from build123d import *

# Parameters (mm, degrees)
F1_DEPTH = 25.4


with BuildPart() as f1:
    # F0 (on Front) → F1 (new body)
    with BuildSketch(Plane.XZ):
        Polygon((47.539182, 77.96976), (47.539182, 65.957407), (47.539182, 61.33727), (47.539182, 53.945053), (91.276467, 53.945053), (91.276467, 77.96976), align=None)
        with BuildLine():
            Line((-2.96659, 32.384418), (-2.96659, 19.140026))
            Line((-2.96659, 19.140026), (15.205946, 19.140026))
            Line((15.205946, 19.140026), (15.205946, 42.856727))
            ThreePointArc((15.205946, 42.856727), (26.010861, 61.477741), (47.539182, 61.33727))
            Line((47.539182, 61.33727), (47.539182, 65.957407))
            ThreePointArc((47.539182, 65.957407), (13.287985, 62.707588), (-2.96659, 32.384418))
        make_face()
        Polygon((-2.96659, 19.140026), (-31.311143, 19.140026), (-31.311143, -19.140026), (31.311143, -19.140026), (31.311143, 19.140026), (15.205946, 19.140026), align=None)
    extrude(amount=F1_DEPTH)


solid = f1.part
Could you check a few things on this model? Use its own coordinates, in mm. A direction names the side the tool comes from. Round coordinates to 2 decimals unless told otherwise and drop trailing zeros. Order: outer loops, then holes, each group sorted by start corner. A loop starts at its lowest first (then second) coordinate and runs counter-clockwise, first axis right, second up.
(1) Please list where these lines run through material, in increasing order: line 1 along Z through (x, y) = (-15.5, -6.5); line 2 along X through (y, z) = (-19.75, 11.5); line 3 along Z through (x, y) = (28, -8.5).
Response values:
line 1: z = -19.14 to 19.14
line 2: x = -31.31 to 31.31
line 3: z = -19.14 to 19.14, 62.48 to 68.39
(2) If we mould it in two halves opening along X, with no side actions, what happens to faces 6 (the flat face through (-31.311, -13, 0)), 7 (the flat face through (-17, -13, 19.14)), 8 (the cylindrical face through (13.708, -12.522, 62.982)), 9 (the flat face through (47.539, -13, 72))? For each: released by +X, released by -X, zero draft, split by the parting line, or undercut.
Response values:
face 6: released by -X
face 7: zero draft
face 8: undercut
face 9: undercut
(3) Imagine slicing it at D-D (x = 53.5). Write out the boundary of the cut face in (y, z).
Response values:
outline: (-25.4, 53.95) - (0, 53.95) - (0, 77.97) - (-25.4, 77.97) - close
(4) Imagine slicing it at C-C (z = 55.5). Write out the boundary of the cut face in (x, y).
Response values:
outline: (5.31, -25.4) - (19.33, -25.4) - (19.33, 0) - (5.31, 0) - close; (47.54, -25.4) - (91.28, -25.4) - (91.28, 0) - (47.54, 0) - close
(5) I'm going to push flat-ended pins straight in: pin 1 (1 mm diameter, centred on x = 34, y = -5.5, fed in from +Z); pin 2 (7.5 mm diameter, centred on x = -24, y = -8.5, fed in from +Z); pin 3 (4 mm diameter, centred on y = -15, z = 27.5, fed in from -X); pin 4 (12 mm diameter, centred on x = 2, z = 7.5, fed in from +Y). Where does each tip first touch, or does it pass through?
Response values:
pin 1: stops at z = 68.8
pin 2: stops at z = 19.14
pin 3: stops at x = -2.97
pin 4: stops at y = 0
(6) Imagine slicing it at B-B (x = 28). Write out the boundary of the cut face in (y, z), plus the area to 3 significant figures.
Response values:
outline: (-25.4, -19.14) - (0, -19.14) - (0, 19.14) - (-25.4, 19.14) - close; (-25.4, 62.48) - (0, 62.48) - (0, 68.39) - (-25.4, 68.39) - close
area: 1,120 mm2
(7) Which directions (+Z, -Z, +X, -X, +Y, -Y) give clear straight access to the entire face, cutting with the end or side of a thin tool? Please do faces 1 (the cylindrical face through (25.74, -12.52, 61.32)), 2 (the flat face through (-2.967, -13, 26)), 3 (the flat face through (23, -13, 19.14)), 4 (the flat face through (69, -13, 53.945)), 5 (the flat face through (47.539, -13, 58)).
Response values:
face 1: +Y, -Y
face 2: +Z, -X, +Y, -Y
face 3: +X, +Y, -Y
face 4: -Z, +X, +Y, -Y
face 5: -Z, +Y, -Y
(8) Imagine slicing it at A-A (y = -7). Write out the boundary of the cut face in (x, z), plus the area to 3 significant figures.
Response values:
outline: (-31.31, -19.14) - (31.31, -19.14) - (31.31, 19.14) - (15.21, 19.14) - (15.21, 42.86) arc R21.45 cw to (47.54, 61.34) - (47.54, 53.95) - (91.28, 53.95) - (91.28, 77.97) - (47.54, 77.97) - (47.54, 65.96) arc R36.41 ccw to (-2.97, 32.38) - (-2.97, 19.14) - (-31.31, 19.14) - close
area: 4,310 mm2
